```python
from build123d import *

# Parameters (mm, degrees)
CYLINDER001_R     = 2.4
CYLINDER001_DEPTH = 10
ARRAY_X_COUNT     = 2
ARRAY_X_PITCH     = 34
ARRAY_Y_COUNT     = 2
ARRAY_Y_PITCH     = 34
TORUS_R           = 1.5
BOX_W             = 40
BOX_H             = 40
BOX_DEPTH         = 4
CYLINDER_R        = 17
CYLINDER_DEPTH    = 50
FILLET_R          = 1


with BuildPart() as taladros:
    # Cylinder001 → Cylinder001 (new body)
    with BuildSketch(Plane(origin=(3, 3, -1), x_dir=(1, 0, 0), z_dir=(0, 0, 1))):
        Circle(CYLINDER001_R)
    extrude(amount=CYLINDER001_DEPTH)

    # Array X: Taladros ×2


with BuildPart() as taladros_1:
    add(taladros.part)
    with Locations(*[(i * ARRAY_X_PITCH, 0, 0) for i in range(1, ARRAY_X_COUNT)]):
        add(taladros.part)

    # Array Y: Taladros ×2


with BuildPart() as taladros_2:
    add(taladros_1.part)
    with Locations(*[(0, i * ARRAY_Y_PITCH, 0) for i in range(1, ARRAY_Y_COUNT)]):
        add(taladros_1.part)


with BuildPart() as obj1:
    # Torus → Torus (revolve)
    with BuildSketch(Plane(origin=(20, 20, 50), x_dir=(1, 0, 0), z_dir=(0, -1, 0))):
        with Locations((10.5, 0)):
            Circle(TORUS_R)
    revolve(axis=Axis((20, 20, 50), (0, 0, 1)))


with BuildPart() as base:
    # Box → Box (new body)
    with BuildSketch(Plane.XY):
        with Locations((20, 20)):
            Rectangle(BOX_W, BOX_H)
    extrude(amount=BOX_DEPTH)


with BuildPart() as obj2:
    # Cylinder → Cylinder (new body)
    with BuildSketch(Plane(origin=(20, 20, 0), x_dir=(1, 0, 0), z_dir=(0, 0, 1))):
        Circle(CYLINDER_R)
    extrude(amount=CYLINDER_DEPTH)

    # Fusion: union Base
    add(base.part)

    # Cut: cut obj1
    add(obj1.part, mode=Mode.SUBTRACT)

    # Cut001: cut Taladros
    add(taladros_2.part, mode=Mode.SUBTRACT)

    # Fillet
    fillet_edges = [obj2.edges().sort_by_distance(p)[0] for p in [
        (3, 20, 50),
        (0, 0, 2),
        (0, 40, 2),
        (40, 40, 2),
        (40, 0, 2),
    ]]
    fillet(fillet_edges, radius=FILLET_R)


solid = obj2.part
```
Could you check a few things on this model? Use its own coordinates, in mm. A direction names the side the tool comes from. Coordinates: 2 decimals unless noted, no trailing zeros. Write each loop counter-clockwise with the first axis right and the second up, starting at its lowest first coordinate (ties: lowest second). Pieces come first, ordered by that corner, then holes. Notation, with made-up numbers: M 47,19.5 L 65,19.5 A13 ccw 65,36.5 Z; hole C 51,-33 d2. An arc over 180 degrees is marked long. Answer as CSV lines item,"result". Start each with the question number.
1) For faces 1 (the cylindrical face through (2.69, 5.38, 1.97)), 2 (the flat face through (19.7, 2.5, 4)), which set-ups out of +Z, -Z, +X, -X, +Y, -Y let a thin tool reach every point of the face, with its end or its side?
2) Please list where these lines run through material, in increasing order: line 1 (Y direction, x = 3, z = 2.4); line 2 (Z direction, x = 2.5, y = 26). Write a range as from..to.
3) For P1, Ø1, axis at x = 14.5, z = 31, coming from the -Y side; P2, Ø1, axis at y = 12.5, z = 24, coming from the +X side; P3, Ø6, axis at x = 37, y = 3, coming from the +Z side, each with a flat end and sliding along its axis, tell me the tip position at first contact or that it passes through.
4) I want a section at C-C, the plane z = 27. Please give me the cut outline in (x, y).
5) I want a section at A-A, the plane y = 20. Please give me the cut outline in (x, z), and give its area (3 significant figures).
6) We'd pull the mould along Y, two halves only. Please class faces 3 (the flat face through (40, 20, 2)), 4 (the cylindrical face through (6.509, 9.656, 26.185)), 5 (the cylindrical face through (2.48, 34.657, 1.972)): +Y half, -Y half, draft (parallel to the pull), parting line (faces both ways), or undercut.
Data:
1,face 1,"+Z, -Z"
1,face 2,"+Z"
2,line 1,"y = 0..0.6, 5.4..34.6, 39.4..40"
2,line 2,"z = 0..4"
3,P1,"stops at y = 3.75"
3,P2,"stops at x = 35.49"
3,P3,"stops at z = 4"
4,outline,"C 20,20 d34"
5,outline,"M 0,0 L 40,0 L 40,4 L 37,4 L 37,49 A1 ccw 36,50 L 32,50 A1.5 cw 29,50 L 11,50 A1.5 cw 8,50 L 4,50 A1 ccw 3,49 L 3,4 L 0,4 Z"
5,area,"1,720 mm^2"
6,face 3,"draft"
6,face 4,"parting line"
6,face 5,"undercut"
